Work out the finished part from the listing and answer in its coordinate system (mm). Coordinates: 2 decimals unless noted, no trailing zeros. Order: outer loops, then holes, each group sorted by start corner. A loop starts at its lowest first (then second) coordinate and runs counter-clockwise, first axis right, second up. Notation, with made-up numbers: M -27,-29.75 L -16,-29.75 A31 ccw -16,9.25 Z; hole C 48.5,13 d8. An arc over 180 degrees is marked long. Answer in a Markdown table with one row per item. Add a question column.
Item 1: The part is cut by section B-B (x = 0). Write down the section's boundary in (y, z) (3 decimals), then the cut area to 3 significant figures.
Item 2: The part is cut by section D-D (z = 2.3). Write down the section's boundary in (x, y), then the cut area to 3 significant figures.
Item 3: The part is cut by section A-A (z = 1.3). Write down the section's boundary in (x, y) (3 decimals), then the cut area to 3 significant figures.
Item 4: The mould has two halves that part along X. Classify faces 1 (the face through (-2.2, 0.6, 1.5)), 2 (the face through (2.485, 0, 1)), 3 (the face through (0, -0.4, 1.02)): released by +X, released by -X, zero draft, split by the parting line, or undercut.
Item 5: Flat-ended cylindrical pins translate along their axes: pin 1 Ø1 at (x, y) = (0.5, 1.5) entering from -Z; pin 2 Ø1 at (y, z) = (0.5, 2.5) entering from +X; pin 3 Ø1 at (x, z) = (1.5, 3) entering from -Y. Find the tip coordinate at first contact, or state that the pin passes through.
Item 6: Consider line 1 (Z direction, x = -1.75, y = -0.4); line 2 (Z direction, x = 2.25, y = 1.7); line 3 (Y direction, x = -1.7, z = 3.1). Determine where each line is inside the solid, lowest interval first. Write a range as from..to.
Autodesk Inventor part; units mm, degrees
ref_plane "YZ Plane" through (0, 0, 0) normal (1, 0, 0) x (0, 1, 0)
ref_plane "XZ Plane" through (0, 0, 0) normal (0, 1, 0) x (-1, 0, 0)
ref_plane "XY Plane" through (0, 0, 0) normal (0, 0, 1) x (1, 0, 0)
sketch "Sketch1" plane through (0, 0, 0) normal (0, 0, 1) x (1, 0, 0)
  line L0 (2.485, 2.485) -> (-2.485, 2.485)
  line L1 (-2.485, 2.485) -> (-2.485, -2.485)
  line L2 (-2.485, -2.485) -> (2.485, -2.485)
  line L3 (2.485, -2.485) -> (2.485, 2.485)
  line L4 (2.485, 2.485) -> (-2.485, -2.485) construction
  line L5 (-2.485, 2.485) -> (2.485, -2.485) construction
  point P0 (0, 0)
  dimension "d0" = 4.97
extrude "Extrusion1" add sketch "Sketch1" along normal blind 1.5
sketch "Sketch2" plane through (0, 0, 1.5) normal (0, 0, 1) x (1, 0, 0)
  circle A0 centre (0, 0) radius 2.1
  dimension "d3" = 4.2
extrude "Extrusion2" add sketch "Sketch2" along normal blind 2.52
sketch "Sketch3" plane through (0, 0, 4.02) normal (0, 0, 1) x (1, 0, 0)
  circle A0 centre (0, 0) radius 2.1
  circle A1 centre (0, 0) radius 0.25
  circle A2 centre (0, 0) radius 2
  dimension "d6" = 0.5
  dimension "d7" = 4
extrude "Extrusion3" cut sketch "Sketch3" against normal blind 3 contours A2
properties part number "Connector" material "Gold"
Reply:
| question | item | result |
|---|---|---|
| 1 | outline | M -2.485,0 L 2.485,0 L 2.485,1.5 L 2.1,1.5 L 2.1,4.02 L 2,4.02 L 2,1.02 L 0.25,1.02 L 0.25,4.02 L -0.25,4.02 L -0.25,1.02 L -2,1.02 L -2,4.02 L -2.1,4.02 L -2.1,1.5 L -2.485,1.5 Z |
| 1 | area | 7.54 mm2 |
| 2 | outline | C 0,0 d4.2; C 0,0 d0.5; hole C 0,0 d4 |
| 2 | area | 1.48 mm2 |
| 3 | outline | M -2.485,-2.485 L 2.485,-2.485 L 2.485,2.485 L -2.485,2.485 Z; C 0,0 d0.5; hole C 0,0 d4 |
| 3 | area | 12.3 mm2 |
| 4 | face 1 | zero draft |
| 4 | face 2 | released by +X |
| 4 | face 3 | undercut |
| 5 | pin 1 | stops at z = 0 |
| 5 | pin 2 | stops at x = 2.1 |
| 5 | pin 3 | stops at y = -1.85 |
| 6 | line 1 | z = 0..1.02 |
| 6 | line 2 | z = 0..1.5 |
| 6 | line 3 | y = -1.23..-1.05, 1.05..1.23 |
